Job drawing, mm, ordinate dimensions from the low corner. One solid piece. Give positions to 0.01 mm unless a question says otherwise; leave off trailing zeros. Loops run counter-clockwise (first coordinate to the right, second up) from the corner with the lowest first, then second, coordinate; pieces in that order, holes last. Notation, with made-up numbers: M 74,33 L 121,33 A15 ccw 121,46 Z; hole C 35.25,65 d5. An arc over 180 degrees is marked long. Answer as CSV lines item,"result".
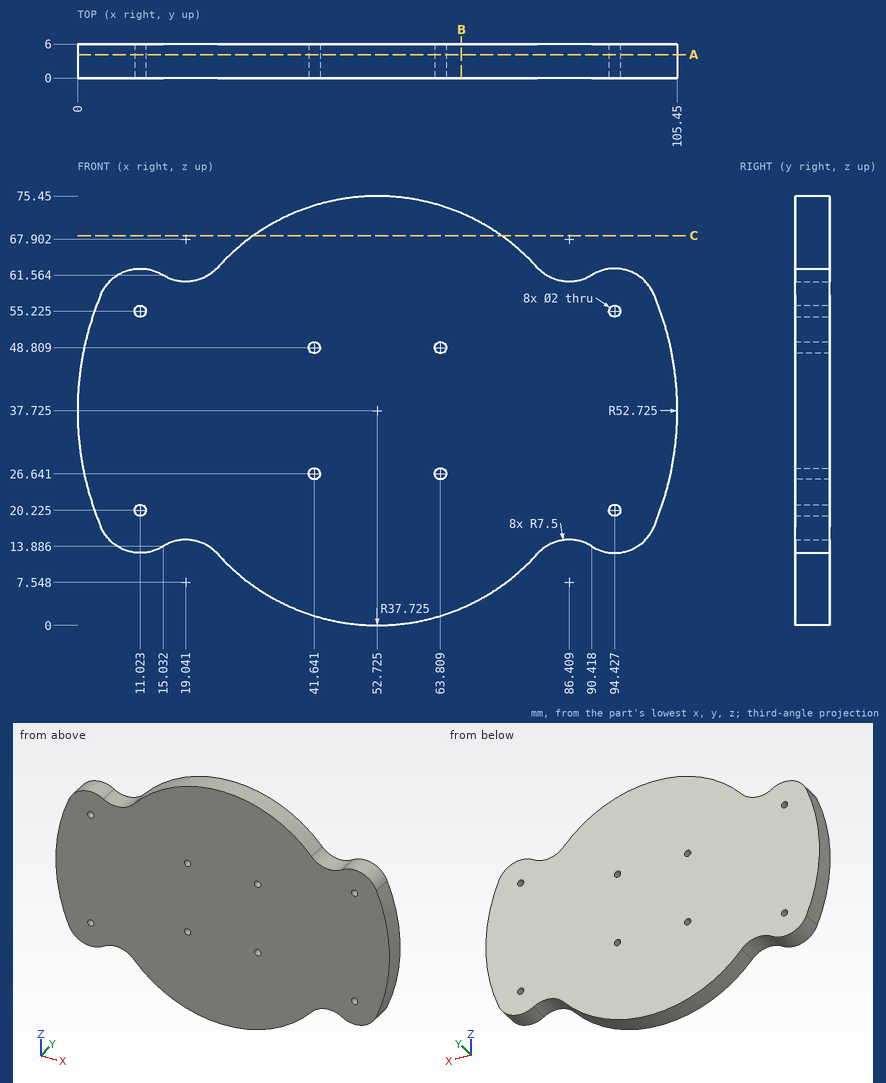
1) Band-saw the part on C-C on z = 68.5. Give the cut face in (x, y), and give its area (3 significant figures).
Answer below:
outline,"M 30.91,0 L 74.54,0 L 74.54,6 L 30.91,6 Z"
area,"262 mm^2"
2) Band-saw the part on A-A on y = 4.15. Give the number of separate pieces and of enclosed holes in the cut face, and give its area (3 significant figures).
Answer below:
separate pieces,"1"
enclosed holes,"8"
area,"5,950 mm^2"
3) Band-saw the part on B-B on x = 67.5. Give the cut face in (y, z).
Answer below:
outline,"M 0,3.01 L 6,3.01 L 6,72.44 L 0,72.44 Z"
4) Drill centre lines: line 1 (Z direction, x = 64, y = 3.7) (1 decimal); line 2 (X direction, y = 4.6, z = 55.5) (1 decimal); line 3 (X direction, y = 2.1, z = 56) (1 decimal). Where is each one in solid material? Low to high. Write a range as from..to.
Answer below:
line 1,"z = 1.7..25.7, 27.6..47.8, 49.8..73.7"
line 2,"x = 3.1..10.1, 12..93.5, 95.4..102.4"
line 3,"x = 3.3..10.4, 11.7..93.8, 95.1..102.2"
5) Flat gauge pins, fed straight in: pin 1 (1.5 mm diameter, centred on x = 40.5, y = 4, fed in from +Z); pin 2 (3 mm diameter, centred on x = 56, y = 1.5, fed in from +Z); pin 3 (2 mm diameter, centred on y = 4, z = 28.5, fed in from +X) (1 decimal); pin 4 (2.5 mm diameter, centred on x = 63.81, z = 48.81, fed in from +Y). Where does each tip first touch, or does it go through?
Answer below:
pin 1,"stops at z = 73.66"
pin 2,"stops at z = 75.41"
pin 3,"stops at x = 104.8"
pin 4,"stops at y = 6"
